Could you check a few things on this model? Use its own coordinates, in mm. Round coordinates to 2 decimals unless told otherwise and drop trailing zeros. Write each loop counter-clockwise with the first axis right and the second up, starting at its lowest first coordinate (ties: lowest second). Pieces come first, ordered by that corner, then holes. Notation, with made-up numbers: (-23.75, 63.5) -> (8.25, 63.5) arc R11 ccw to (8.25, 74.5) -> close; hole circle Ø8 at (-9, -14.5). An arc over 180 degrees is marked (long way). Answer in a Markdown table with one row per item.
from build123d import *

# Parameters (mm, degrees)
CUT_EXTRUDE_1_DEPTH = 0.65


with BuildPart() as part:
    # 草图1 → 旋转1 (revolve)
    with BuildSketch(Plane(origin=(0, 0, 0), x_dir=(0, 0, -1), z_dir=(1, 0, 0))):
        with BuildLine():
            Line((0, 0), (0, 0.9))
            ThreePointArc((0, 0.9), (0.633393287, 1.544344521), (1.5, 1.8))
            Line((1.5, 1.8), (1.5, 1))
            Line((1.5, 1), (11.5, 1))
            Line((11.5, 1), (11.5, 0))
            Line((11.5, 0), (0, 0))
        make_face()
    revolve(axis=Axis((0, 0, 0), (0, 0, 1)))

    # 草图2 → 切除-拉伸1 (cut)
    with BuildSketch(Plane.XY):
        Polygon((0.75055535, 0), (0.375277675, 0.65), (-0.375277675, 0.65), (-0.75055535, 0), (-0.375277675, -0.65), (0.375277675, -0.65), align=None)
    extrude(amount=-CUT_EXTRUDE_1_DEPTH, mode=Mode.SUBTRACT)


solid = part.part
1) Please list where these lines run through material, in increasing order: line 1 (Z direction, x = -0.25, y = -0.35); line 2 (X direction, y = -0.5, z = -5.25); line 3 (Z direction, x = 0.05, y = 1.1).
Findings:
| item | result |
|---|---|
| line 1 | z = -11.5 to -0.65 |
| line 2 | x = -0.87 to 0.87 |
| line 3 | z = -1.5 to -0.13 |
2) Thinking about a two-plate mould opening in X: for faces 1 (the face through (1, 0, -7)), 2 (the face through (0, 0, -0.65)), 3 (the face through (1, 1, -1.5)), which applies, +X half, -X half, draft (parallel to the pull), parting line (faces both ways), or undercut?
Findings:
| item | result |
|---|---|
| face 1 | parting line |
| face 2 | undercut |
| face 3 | draft |
3) Imagine slicing it at B-B, the plane z = -5.5. Please give me the cut outline in (x, y).
Findings:
| item | result |
|---|---|
| outline | circle Ø2 at (0, 0) |
4) For pin 1 (1 mm diameter, centred on x = 0, y = -0.5, fed in from +Z); pin 2 (2 mm diameter, centred on y = 1, z = -6.5, fed in from -X); pin 3 (0.7 mm diameter, centred on x = 0, z = -0.5, fed in from +Y), each with a flat end and sliding along its axis, tell me the tip position at first contact or that it passes through.
Findings:
| item | result |
|---|---|
| pin 1 | stops at z = 0 |
| pin 2 | stops at x = -1 |
| pin 3 | stops at y = 1.66 |
5) Imagine slicing it at A-A, the plane x = 0. Please give me the cut outline in (y, z).
Findings:
| item | result |
|---|---|
| outline | (-1.8, -1.5) -> (-1, -1.5) -> (-1, -11.5) -> (1, -11.5) -> (1, -1.5) -> (1.8, -1.5) arc R1.8 ccw to (0.9, 0) -> (0.65, 0) -> (0.65, -0.65) -> (-0.65, -0.65) -> (-0.65, 0) -> (-0.9, 0) arc R1.8 ccw to start |
